The listing builds one solid part. Answer for the finished solid, in the listing's coordinates (mm). A direction names the side the tool comes from. Round coordinates to 2 decimals unless told otherwise and drop trailing zeros. Write each loop counter-clockwise with the first axis right and the second up, starting at its lowest first coordinate (ties: lowest second). Pieces come first, ordered by that corner, then holes.
from build123d import *

# Parameters (mm, degrees)
AUFSATZ_LINEAR_AUSTRAGEN2_DEPTH = 1.5
AUFSATZ_LINEAR_AUSTRAGEN3_DEPTH = 1.5


with BuildPart() as part:
    # Skizze1 → Aufsatz-Linear austragen2 (new body)
    with BuildSketch(Plane(origin=(0, 0, 0), x_dir=(1, 0, 0), z_dir=(0, 1, 0))):
        with BuildLine():
            Line((-126.5, 0), (126.5, 0))
            ThreePointArc((126.5, 0), (0, 126.5), (-126.5, 0))
        make_face()
    extrude(amount=AUFSATZ_LINEAR_AUSTRAGEN2_DEPTH)

    # Skizze2 → Aufsatz-Linear austragen3 (add)
    with BuildSketch(Plane.XY):
        Polygon((126.5, 0), (147, 90), (-147, 90), (-126.5, 0), align=None)
    extrude(amount=AUFSATZ_LINEAR_AUSTRAGEN3_DEPTH)


solid = part.part
1. A straight line is drawn through the part: line 1 along Y through (x, z) = (-22, -10). Find the intervals that lie inside material, in ascending order.
Geometry says:
line 1: y = 0 to 1.5
2. Given pin 1 (2 mm diameter, centred on x = -25.5, y = 12, fed in from -Z), flat-ended and moving along its own axis, determine where the tip first touches the part or whether it passes through.
Geometry says:
pin 1: stops at z = 0
3. Section D-D on x = 120 is taken. Determine the outline of the cut face in (y, z), plus the area to 3 significant figures.
Geometry says:
outline: (0, -40.03) - (1.5, -40.03) - (1.5, 0) - (90, 0) - (90, 1.5) - (0, 1.5) - close
area: 195 mm2
4. Section C-C on z = -54.5 is taken. Determine the outline of the cut face in (x, y).
Geometry says:
outline: (-114.16, 0) - (114.16, 0) - (114.16, 1.5) - (-114.16, 1.5) - close
5. A tool of negligible diameter and unlimited length cuts with its end or side. For faces 1 (the face through (-136.894, 45.63, 0.74)), 2 (the face through (-2, 46, 0)), from which of +Z, -Z, +X, -X, +Y, -Y can it reach the whole face along a straight path? Write none if from no direction.
Geometry says:
face 1: +Z, -Z, -X, -Y
face 2: -Z, +X, -X, +Y
6. Section B-B on y = 17 is taken. Determine the outline of the cut face in (x, z), plus the area to 3 significant figures.
Geometry says:
outline: (-130.37, 0) - (130.37, 0) - (130.37, 1.5) - (-130.37, 1.5) - close
area: 391 mm2
7. Section A-A on x = 0 is taken. Determine the outline of the cut face in (y, z).
Geometry says:
outline: (0, -126.5) - (1.5, -126.5) - (1.5, 0) - (90, 0) - (90, 1.5) - (0, 1.5) - close
